Source: CAD feature listing. Evaluate the final solid. Frame: model axes, mm. Face numbers are marked on the shaded views. A direction names the side the tool comes from. Round coordinates to 2 decimals unless told otherwise and drop trailing zeros. Loops run counter-clockwise (first coordinate to the right, second up) from the corner with the lowest first, then second, coordinate; pieces in that order, holes last. Notation, with made-up numbers: M 79.5,75.25 L 84.5,75.25 A27 ccw 84.5,107.25 Z; hole C -22,-27.5 d2. An arc over 180 degrees is marked long. Write each question's results on one line, items separated by ' | '. Start each with the question number.
1. Section A-A on y = 23. Output: boundary loops of the cut face in (x, z).
2. Section B-B on z = 20.5. Output: boundary loops of the cut face in (x, y).
3. Section C-C on z = 5.08. Give the number of separate pieces and of enclosed holes in the cut face, and give its area (3 significant figures).
4. Ray query, line 1 (Y direction, x = 0.5, z = 15); line 2 (Z direction, x = 29, y = 0); line 3 (X direction, y = 5.5, z = 11). Return the intervals inside material, ascending.
5. Draft query along Y for the marked faces 6, 7, 8 and 9. Return one class per face: released by +Y, released by -Y, zero draft, split by the parting line, or undercut.
6. Set-up query: the marked faces 1, 2, 3, 4 and 5. Return all of +Z, -Z, +X, -X, +Y, -Y with unobstructed straight access to the full face (end or side cutting, diameter ignored); none if empty.
7. Contact query for flat-ended pins moving along their axis: pin 1 Ø4 at (y, z) = (-25.5, 44) entering from +X; pin 2 Ø7 at (x, z) = (0, 5.08) entering from +Y; pin 3 Ø2.5 at (y, z) = (1, 6) entering from -X; pin 4 Ø2.5 at (y, z) = (0, 5.08) entering from +X. Output: stop coordinate, or through.
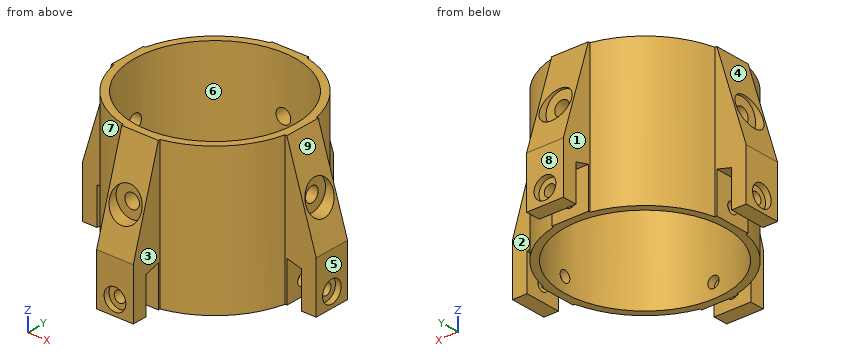
from build123d import *

# Parameters (mm, degrees)
SKETCH3_R         = 30.32125
SKETCH3_R_2       = 27.78125
BASE_RING_DEPTH   = 50.8
HOOK_DEPTH        = 6.35
CIRPATTERN1_COUNT = 4


with BuildPart() as part:
    # Sketch3 → base_ring (new body)
    with BuildSketch(Plane(origin=(0, 0, 0), x_dir=(0, 1, 0), z_dir=(0, 0, 1))):
        with Locations(Location((0, 0, 0), (0, 0, 270))):
            Circle(SKETCH3_R)
        with Locations(Location((0, 0, 0), (0, 0, 270))):
            Circle(SKETCH3_R_2, mode=Mode.SUBTRACT)
    extrude(amount=BASE_RING_DEPTH)

    # Sketch6 → hook (add, symmetric)
    with BuildSketch(Plane.YZ):
        Polygon((27.78125, 50.8), (27.78125, 0), (30.32125, 0), (30.32125, 14.061181898), (35.40125, 12.7), (35.40125, 0), (40.48125, 0), (40.48125, 17.78), (30.32125, 50.8), align=None)
    hook = extrude(amount=HOOK_DEPTH, both=True)

    # Sketch8 → CBORE for #5 Binding Head Machine Screw1 (revolve, cut)
    with BuildSketch(Plane(origin=(0, 40.48125, 5.08), x_dir=(0, 0, 1), z_dir=(1, 0, 0))):
        Polygon((0, 0), (0, 39.275163199), (1.9558, 38.1), (1.9558, 1.9812), (3.77063, 1.9812), (3.77063, 0), align=None)
    cbore_for_5_binding_head_machine_screw1 = revolve(axis=Axis((0, 46.83125, 5.08), (0, -1, 0)), mode=Mode.SUBTRACT)

    # Sketch10 → CBORE for #10 Binding Head Machine Screw2 (revolve, cut)
    with BuildSketch(Plane(origin=(0, 40.48125, 31.75), x_dir=(0, 0, 1), z_dir=(1, 0, 0))):
        Polygon((0, 0), (0, 39.633816902), (2.5527, 38.1), (2.5527, 6.9342), (5.55625, 6.9342), (5.55625, 0), align=None)
    cbore_for_10_binding_head_machine_screw = revolve(axis=Axis((0, 46.83125, 31.75), (0, -1, 0)), mode=Mode.SUBTRACT)

    # CirPattern1: hook, CBORE for #5 Binding Head Machine Screw1, CBORE for #10 Binding Head Machine Screw2 ×4 about axis
    cirpattern1_axis = Axis((0, 0, 0), (0, 0, 1))
    add([hook.rotate(cirpattern1_axis, i * 360 / CIRPATTERN1_COUNT) for i in range(1, CIRPATTERN1_COUNT)])
    add([cbore_for_5_binding_head_machine_screw1.rotate(cirpattern1_axis, i * 360 / CIRPATTERN1_COUNT) for i in range(1, CIRPATTERN1_COUNT)], mode=Mode.SUBTRACT)
    add([cbore_for_10_binding_head_machine_screw.rotate(cirpattern1_axis, i * 360 / CIRPATTERN1_COUNT) for i in range(1, CIRPATTERN1_COUNT)], mode=Mode.SUBTRACT)


solid = part.part
Taken from the geometry:
1) outline: M -19.76,0 L -15.58,0 L -15.58,50.8 L -19.76,50.8 Z; M 15.58,0 L 19.76,0 L 19.76,50.8 L 15.58,50.8 Z
2) outline: M -39.64,-6.35 L -29.65,-6.35 A30.32 ccw -6.35,-29.65 L -6.35,-39.64 L 6.35,-39.64 L 6.35,-29.65 A30.32 ccw 29.65,-6.35 L 39.64,-6.35 L 39.64,6.35 L 29.65,6.35 A30.32 ccw 6.35,29.65 L 6.35,39.64 L -6.35,39.64 L -6.35,29.65 A30.32 ccw -29.65,6.35 L -39.64,6.35 Z; hole C 0,0 d55.56
3) separate pieces: 12 | enclosed holes: 0 | area: 585 mm^2
4) line 1: -40.48 to -27.78, 27.78 to 40.48 | line 2: 0 to 3.12, 7.04 to 29.2, 34.3 to 50.8 | line 3: -40.48 to -35.4, -30.32 to -27.23, 27.23 to 30.32, 35.4 to 40.48
5) face 6: undercut | face 7: released by -Y | face 8: released by +Y | face 9: zero draft
6) face 1: +Z, -Z, -X, +Y | face 2: +Z, -Z, +X, +Y | face 3: +Z, -Z, +X, -Y | face 4: +Z, -X, +Y, -Y | face 5: +Z, -Z, +X, +Y, -Y
7) pin 1: x = 19.16 | pin 2: y = 38.5 | pin 3: x = -38.5 | pin 4: through
